The figure shows three views and two pictorial views of one solid part (mm, origin at its lowest corner). Answer the questions. A direction names the side the tool comes from. Round coordinates to 2 decimals unless told otherwise and drop trailing zeros. Order: outer loops, then holes, each group sorted by start corner. A loop starts at its lowest first (then second) coordinate and runs counter-clockwise, first axis right, second up. Notation, with made-up numbers: (9.5, -39.5) -> (32.5, -39.5) arc R22 ccw to (32.5, -33.5) -> close; hole circle Ø3 at (-15.5, 28.5). An arc over 180 degrees is marked (long way). One line per item, written item: value. Start each with the question number.
1. Section D-D (y = 66.5) is taken. Give the vertices of the cut face in (x, z), then the cut area to 3 significant figures.
2. Section A-A (z = 33) is taken. State how many separate pieces and enclosed holes the cut face has, then the cut area to 3 significant figures.
3. Consider line 1 (X direction, y = 5, z = 45); line 2 (X direction, y = 19, z = 33); line 3 (X direction, y = 46, z = 6.5). Determine where each line is inside the solid, lowest interval first.
4. For the marked faces 4, 5, 6 and 7, determine the directions among +Z, -Z, +X, -X, +Y, -Y from which every point of the face is accessible in a straight line to the end or side of a thin tool.
5. Section B-B (x = 22.5) is taken. Give the vertices of the cut face in (y, z).
6. Flat-ended cylindrical pins translate along their axes: pin 1 Ø12 at (y, z) = (64.5, 41) entering from -X; pin 2 Ø3 at (y, z) = (5.5, 19) entering from -X; pin 3 Ø10 at (x, z) = (91.5, 15.5) entering from +Y; pin 4 Ø16 at (x, z) = (185, 30.5) entering from +Y. Find the tip coordinate at first contact, or state that the pin passes through.
7. Section C-C (y = 5) is taken. Give the vertices of the cut face in (x, z), then the cut area to 3 significant figures.
8. The mould has two halves that part along X. Classify the marked faces 1, 2 and 3: released by +X, released by -X, zero draft, split by the parting line, or undercut.
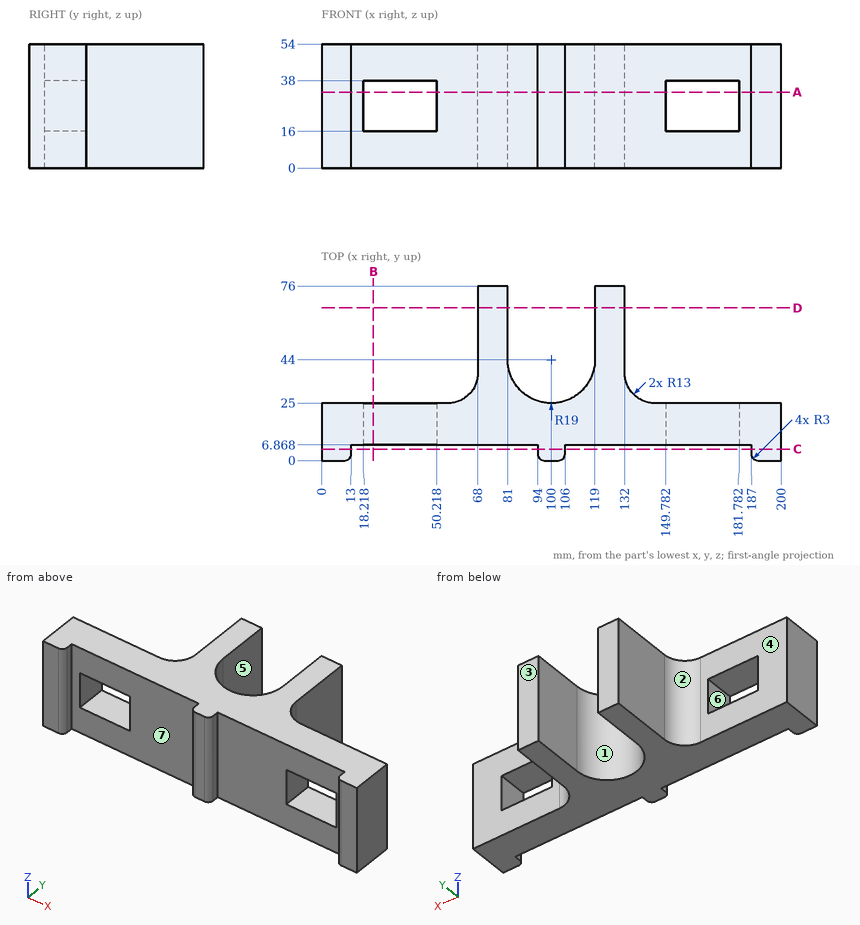
Answer:
1. outline: (68, 0) -> (81, 0) -> (81, 54) -> (68, 54) -> close; (119, 0) -> (132, 0) -> (132, 54) -> (119, 54) -> close
1. area: 1,400 mm^2
2. separate pieces: 3
2. enclosed holes: 0
2. area: 4,270 mm^2
3. line 1: 0 to 13, 94 to 106, 187 to 200
3. line 2: 0 to 18.22, 50.22 to 149.78, 181.78 to 200
3. line 3: 68 to 81, 119 to 132
4. face 4: +Z, -Z, -X, +Y
4. face 5: +Z, -Z, +Y
4. face 6: +Y, -Y
4. face 7: +Z, -Z, -Y
5. outline: (6.87, 0) -> (25, 0) -> (25, 16) -> (6.87, 16) -> close; (6.87, 38) -> (25, 38) -> (25, 54) -> (6.87, 54) -> close
6. pin 1: x = 68
6. pin 2: x = 0
6. pin 3: y = 30.63
6. pin 4: y = 25
7. outline: (0, 0) -> (13, 0) -> (13, 54) -> (0, 54) -> close; (94, 0) -> (106, 0) -> (106, 54) -> (94, 54) -> close; (187, 0) -> (200, 0) -> (200, 54) -> (187, 54) -> close
7. area: 2,050 mm^2
8. face 1: undercut
8. face 2: released by -X
8. face 3: zero draft
